```python
from build123d import *

# Parameters (mm, degrees)
F1_DEPTH = 50


with BuildPart() as f1:
    # F0 (on Front) → F1 (new body)
    with BuildSketch(Plane.XZ):
        with BuildLine():
            Line((91.4418067738, 17.4405043857), (4.1054428346, 24.6606029758))
            ThreePointArc((4.1054428346, 24.6606029758), (19.0740146648, 16.1611251022), (25, 0))
            ThreePointArc((25, 0), (19.0740146648, -16.1611251022), (4.1054428346, -24.6606029758))
            Line((4.1054428346, -24.6606029758), (91.4418067738, -17.4405043857))
            ThreePointArc((91.4418067738, -17.4405043857), (72.5, 0), (91.4418067738, 17.4405043857))
        make_face()
        with BuildLine():
            ThreePointArc((4.1054428346, 24.6606029758), (2.0597239626, 24.9150062653), (0, 25))
            Line((0, 25), (4.1054428346, 24.6606029758))
        make_face()
        with BuildLine():
            Line((4.1054428346, -24.6606029758), (0, -25))
            ThreePointArc((0, -25), (2.0597239626, -24.9150062653), (4.1054428346, -24.6606029758))
        make_face()
        with BuildLine():
            ThreePointArc((107.5, 0), (102.8740362463, 11.8536572723), (91.4418067738, 17.4405043857))
            ThreePointArc((91.4418067738, 17.4405043857), (72.5, 0), (91.4418067738, -17.4405043857))
            ThreePointArc((91.4418067738, -17.4405043857), (102.8740362463, -11.8536572723), (107.5, 0))
        make_face()
        with BuildLine():
            Line((4.1054428346, 24.6606029758), (0, 25))
            ThreePointArc((0, 25), (-25, 0), (0, -25))
            Line((0, -25), (4.1054428346, -24.6606029758))
            ThreePointArc((4.1054428346, -24.6606029758), (19.0740146648, -16.1611251022), (25, 0))
            ThreePointArc((25, 0), (19.0740146648, 16.1611251022), (4.1054428346, 24.6606029758))
        make_face()
    extrude(amount=F1_DEPTH)


solid = f1.part
```
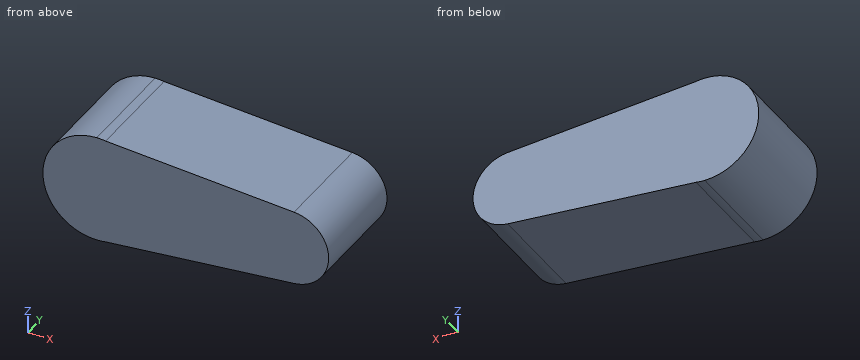
Part model, mm, in its own coordinate system. Round coordinates to 2 decimals unless told otherwise and drop trailing zeros. Order: outer loops, then holes, each group sorted by start corner. A loop starts at its lowest first (then second) coordinate and runs counter-clockwise, first axis right, second up. Notation, with made-up numbers: M -34.75,73.25 L -14.75,73.25 A20 ccw -14.75,86.25 Z; hole C 83,44.25 d9. An arc over 180 degrees is marked long. Answer in a Markdown table with one row per item. Add a question column.
Q1. Cut at A-A on y = -23. Give the cut face in (x, z).
Q2. Pin check, flat tips, straight feed: pin 1 (6 mm diameter, centred on x = 62, y = -39.5, fed in from -Z); pin 2 (8 mm diameter, centred on y = -7.5, z = 17.5, fed in from +X); pin 3 (1 mm diameter, centred on x = 11, y = -9.5, fed in from +Z). Stop position of each tip, or through.
Q3. Wall check: L1, parallel to X at y = -10.5, z = 13; L2, parallel to Z at x = 92, y = -7; L3, parallel to X at y = -36.5, z = 6.5. Give the ranges that are in metal, low to high. Write a range as from..to.
Q4. Cut at C-C on x = 25. Give the cut face in (y, z), and give its area (3 significant figures).
Q5. Cut at B-B on z = -21. Give the cut face in (x, y), and give its area (3 significant figures).
Established:
| question | item | result |
|---|---|---|
| 1 | outline | M 4.11,-24.66 L 91.44,-17.44 A17.5 ccw 91.44,17.44 L 4.11,24.66 A25 ccw long Z |
| 2 | pin 1 | stops at z = -20.12 |
| 2 | pin 2 | stops at x = 101.14 |
| 2 | pin 3 | stops at z = 24.13 |
| 3 | L1 | x = -21.35..101.72 |
| 3 | L2 | z = -17.39..17.39 |
| 3 | L3 | x = -24.14..106.25 |
| 4 | outline | M -50,-22.93 L 0,-22.93 L 0,22.93 L -50,22.93 Z |
| 4 | area | 2,290 mm2 |
| 5 | outline | M -13.56,-50 L 48.39,-50 L 48.39,0 L -13.56,0 Z |
| 5 | area | 3,100 mm2 |
